Read the model definition and answer for the solid it produces. Units are mm, in the model's axes. A direction names the side the tool comes from. Round coordinates to 2 decimals unless told otherwise and drop trailing zeros. Write each loop counter-clockwise with the first axis right and the second up, starting at its lowest first coordinate (ties: lowest second). Pieces come first, ordered by that corner, then holes. Notation, with made-up numbers: (39.5, 42.25) -> (74.5, 42.25) arc R25 cw to (74.5, 75.25) -> close; hole circle Ø6 at (8, 88.5). An arc over 180 degrees is marked (long way). Return JSON: item names as keys, results as strings. Group by question number.
(1) The mould has two halves that part along Y. Classify faces 1 (the flat face through (10.5, -14.92, -116.85)), 2 (the cylindrical face through (-1.66, -13.85, -57.61)), 3 (the conical face through (4.16, -1.26, 25.87)): released by +Y, released by -Y, zero draft, split by the parting line, or undercut.
(2) For faces 4 (the flat face through (0, 0, 42.205)), 5 (the flat face through (-2, 16, -115.91)), 6 (the cylindrical face through (-21.714, 10.874, -116.876)), determine the directions among +Z, -Z, +X, -X, +Y, -Y from which every point of the face is accessible in a straight line to the end or side of a thin tool.
(3) Straight lines are drawn through the part: line 1 (Z direction, x = 1, y = 0.5); line 2 (Y direction, x = 2, z = 27); line 3 (Y direction, x = 11, z = -31). For each, find the intervals that lie inside material, in ascending order.
(4) A cutting plane is placed at A-A on z = -40.5. Give the vertices of the cut face in (x, y) (3 decimals), then the cut area to 3 significant figures.
(5) Given pin 1 (5 mm diameter, centred on y = -14, z = -89, fed in from -X); pin 2 (2 mm diameter, centred on x = 8, z = -14.5, fed in from -Y); pin 3 (2 mm diameter, centred on y = 5.5, z = -45.5, fed in from -X), each flat-ended and moving along its own axis, determine where each tip first touches the part or whether it passes through.
```python
from build123d import *

# Parameters (mm, degrees)
FILLET1_R           = 3.81
SHELL1_T            = -1.905
BOSS_EXTRUDE1_START = -1.905
SKETCH2_R           = 15.875
BOSS_EXTRUDE1_DEPTH = 1.905
FILLET2_R           = 3.81
FILLET3_R           = 1.27


with BuildPart() as part:
    # Sketch1 → Revolve1 (revolve)
    with BuildSketch(Plane(origin=(0, 0, 0), x_dir=(1, 0, 0), z_dir=(0, 1, 0))):
        Polygon((16.038285714, 117.815178571), (16.038285714, -2.631621429), (5.497285714, -3.901621429), (3.401785714, -44.109821429), (0.163285714, -44.109821429), (0.163285714, 117.815178571), align=None)
    revolve(axis=Axis((0.163285714, 0, 44.109821429), (0, 0, -1)))

    # Fillet1
    fillet1_edges = [part.edges().sort_by_distance(p)[0] for p in [
        (-5.170714286, 0, 3.901621429),
    ]]
    fillet(fillet1_edges, radius=FILLET1_R)

    # Shell1
    shell1_openings = [part.faces().sort_by_distance(p)[0] for p in [
        (0.163285714, 0, -117.815178571),
    ]]
    offset(amount=SHELL1_T, openings=shell1_openings, kind=Kind.INTERSECTION)

    # Sketch2 → Boss-Extrude1 (add)
    with BuildSketch(Plane(origin=(0, 0, -117.815178571), x_dir=(-1, 0, 0), z_dir=(0, 0, -1)).offset(BOSS_EXTRUDE1_START)):
        Polygon((-0.163285714, 17.8435), (22.506214286, 11.43), (22.506214286, -11.43), (-0.163285714, -17.8435), (-22.832785714, -11.43), (-22.832785714, 11.43), align=None)
        with Locations((-0.163285714, 0)):
            Circle(SKETCH2_R, mode=Mode.SUBTRACT)
    extrude(amount=BOSS_EXTRUDE1_DEPTH)

    # Fillet2
    fillet2_edges = [part.edges().sort_by_distance(p)[0] for p in [
        (0.163285714, 17.8435, -116.862678571),
        (-22.506214286, 11.43, -116.862678571),
        (-22.506214286, -11.43, -116.862678571),
        (0.163285714, -17.8435, -116.862678571),
        (22.832785714, -11.43, -116.862678571),
        (22.832785714, 11.43, -116.862678571),
    ]]
    fillet(fillet2_edges, radius=FILLET2_R)

    # Fillet3
    fillet3_edges = [part.edges().sort_by_distance(p)[0] for p in [
        (-15.711714286, 0, 2.631621429),
    ]]
    fillet(fillet3_edges, radius=FILLET3_R)


solid = part.part
```
Checks:
{
 "1": {"face 1": "released by -Y", "face 2": "undercut", "face 3": "split by the parting line"},
 "2": {"face 4": "-Z", "face 5": "+Z", "face 6": "+Z, -Z, -X, +Y"},
 "3": {"line 1": "z = 42.2 to 44.11", "line 2": "y = -3.7 to -1.25, 1.25 to 3.7", "line 3": "y = -11.6 to -8.82, 8.82 to 11.6"},
 "4": {"outline": "circle Ø31.75 at (0.163, 0); hole circle Ø27.94 at (0.163, 0)", "area": "179 mm^2"},
 "5": {"pin 1": "stops at x = -10.78", "pin 2": "stops at y = -14.33", "pin 3": "stops at x = -15.06"}
}
